Read the model definition and answer for the solid it produces. Units are mm, in the model's axes. A direction names the side the tool comes from. Coordinates: 2 decimals unless noted, no trailing zeros. Order: outer loops, then holes, each group sorted by start corner. A loop starts at its lowest first (then second) coordinate and runs counter-clockwise, first axis right, second up. Notation, with made-up numbers: (48, 87) - (83, 87) arc R28 cw to (83, 118) - close; hole circle Ø5 at (43.5, 50). An arc over 180 degrees is marked (long way). Write item = value, one per line.
from build123d import *

# Parameters (mm, degrees)
SKETCH1_W              = 140
SKETCH1_H              = 35
BOSS_EXTRUDE1_DEPTH    = 6
SKETCH2_R              = 4.5
SKETCH2_R_2            = 5.1
CUT_EXTRUDE1_DEPTH     = 7
CUT_EXTRUDE2_DEPTH     = 7
SKETCH234_W            = 10
SKETCH234_H            = 6
BOSS_EXTRUDE234_DEPTH  = 6
FILLET134_R            = 1
SKETCH2341_W           = 10
SKETCH2341_H           = 6
BOSS_EXTRUDE2341_DEPTH = 6
FILLET1341_R           = 1
SKETCH2342_W           = 10
SKETCH2342_H           = 6
BOSS_EXTRUDE2342_DEPTH = 6
FILLET1342_R           = 1
SKETCH2343_W           = 10
SKETCH2343_H           = 6
BOSS_EXTRUDE2343_DEPTH = 6
FILLET1343_R           = 1
SKETCH2344_W           = 10
SKETCH2344_H           = 6
BOSS_EXTRUDE2344_DEPTH = 6
FILLET1344_R           = 1
SKETCH2345_W           = 10
SKETCH2345_H           = 6
BOSS_EXTRUDE2345_DEPTH = 6
FILLET1345_R           = 1
SKETCH2346_W           = 10
SKETCH2346_H           = 6
BOSS_EXTRUDE2346_DEPTH = 6
FILLET1346_R           = 1
SKETCH2347_W           = 10
SKETCH2347_H           = 6
BOSS_EXTRUDE2347_DEPTH = 6
FILLET1347_R           = 1
SKETCH6_W              = 10
SKETCH6_H              = 6
CUT_EXTRUDE11_DEPTH    = 4
SKETCH61_W             = 10
SKETCH61_H             = 6
CUT_EXTRUDE12_DEPTH    = 4
SKETCH62_W             = 10
SKETCH62_H             = 6
CUT_EXTRUDE13_DEPTH    = 4
FILLET1348_R           = 5


with BuildPart() as part:
    # Sketch1 → Boss-Extrude1 (new body)
    with BuildSketch(Plane(origin=(0, 0, 0), x_dir=(1, 0, 0), z_dir=(0, 1, 0))):
        with Locations((70, 17.5)):
            Rectangle(SKETCH1_W, SKETCH1_H)
    extrude(amount=BOSS_EXTRUDE1_DEPTH)

    # Sketch2 → Cut-Extrude1 (cut, through all)
    with BuildSketch(Plane(origin=(0, 6, 0), x_dir=(1, 0, 0), z_dir=(0, 1, 0))):
        with Locations((66.4, 19)):
            Circle(SKETCH2_R)
        with Locations((35.4, 19)):
            Circle(SKETCH2_R_2)
    extrude(amount=-CUT_EXTRUDE1_DEPTH, mode=Mode.SUBTRACT)

    # Sketch3 → Cut-Extrude2 (cut, through all)
    with BuildSketch(Plane(origin=(0, 6, 0), x_dir=(1, 0, 0), z_dir=(0, 1, 0))):
        Polygon((140, 8), (100, 35), (140, 35), align=None)
    extrude(amount=-CUT_EXTRUDE2_DEPTH, mode=Mode.SUBTRACT)

    # Sketch234 → Boss-Extrude234 (add)
    with BuildSketch(Plane(origin=(119.232221392, 0, 0), x_dir=(1, 0, 0), z_dir=(0, 0, 1))):
        with Locations((0.767778608, 3)):
            Rectangle(SKETCH234_W, SKETCH234_H)
    extrude(amount=BOSS_EXTRUDE234_DEPTH)

    # Fillet134
    fillet134_edges = [part.edges().sort_by_distance(p)[0] for p in [
        (115, 3, 6),
        (125, 3, 6),
    ]]
    fillet(fillet134_edges, radius=FILLET134_R)

    # Sketch2341 → Boss-Extrude2341 (add)
    with BuildSketch(Plane(origin=(85.898888059, 0, 0), x_dir=(1, 0, 0), z_dir=(0, 0, 1))):
        with Locations((0.767778608, 3)):
            Rectangle(SKETCH2341_W, SKETCH2341_H)
    extrude(amount=BOSS_EXTRUDE2341_DEPTH)

    # Fillet1341
    fillet1341_edges = [part.edges().sort_by_distance(p)[0] for p in [
        (91.666666667, 3, 6),
        (81.666666667, 3, 6),
    ]]
    fillet(fillet1341_edges, radius=FILLET1341_R)

    # Sketch2342 → Boss-Extrude2342 (add)
    with BuildSketch(Plane(origin=(52.565554726, 0, 0), x_dir=(1, 0, 0), z_dir=(0, 0, 1))):
        with Locations((0.767778608, 3)):
            Rectangle(SKETCH2342_W, SKETCH2342_H)
    extrude(amount=BOSS_EXTRUDE2342_DEPTH)

    # Fillet1342
    fillet1342_edges = [part.edges().sort_by_distance(p)[0] for p in [
        (58.333333333, 3, 6),
        (48.333333333, 3, 6),
    ]]
    fillet(fillet1342_edges, radius=FILLET1342_R)

    # Sketch2343 → Boss-Extrude2343 (add)
    with BuildSketch(Plane(origin=(19.232221392, 0, 0), x_dir=(1, 0, 0), z_dir=(0, 0, 1))):
        with Locations((0.767778608, 3)):
            Rectangle(SKETCH2343_W, SKETCH2343_H)
    extrude(amount=BOSS_EXTRUDE2343_DEPTH)

    # Fillet1343
    fillet1343_edges = [part.edges().sort_by_distance(p)[0] for p in [
        (25, 3, 6),
        (15, 3, 6),
    ]]
    fillet(fillet1343_edges, radius=FILLET1343_R)

    # Sketch2344 → Boss-Extrude2344 (add)
    with BuildSketch(Plane(origin=(84.232221392, 6, -35), x_dir=(1, 0, 0), z_dir=(0, 0, -1))):
        with Locations((0.767778608, 3)):
            Rectangle(SKETCH2344_W, SKETCH2344_H)
    extrude(amount=BOSS_EXTRUDE2344_DEPTH)

    # Fillet1344
    fillet1344_edges = [part.edges().sort_by_distance(p)[0] for p in [
        (80, 3, -41),
        (90, 3, -41),
    ]]
    fillet(fillet1344_edges, radius=FILLET1344_R)

    # Sketch2345 → Boss-Extrude2345 (add)
    with BuildSketch(Plane(origin=(60.898888059, 6, -35), x_dir=(1, 0, 0), z_dir=(0, 0, -1))):
        with Locations((0.767778608, 3)):
            Rectangle(SKETCH2345_W, SKETCH2345_H)
    extrude(amount=BOSS_EXTRUDE2345_DEPTH)

    # Fillet1345
    fillet1345_edges = [part.edges().sort_by_distance(p)[0] for p in [
        (66.666666667, 3, -41),
        (56.666666667, 3, -41),
    ]]
    fillet(fillet1345_edges, radius=FILLET1345_R)

    # Sketch2346 → Boss-Extrude2346 (add)
    with BuildSketch(Plane(origin=(37.565554726, 6, -35), x_dir=(1, 0, 0), z_dir=(0, 0, -1))):
        with Locations((0.767778608, 3)):
            Rectangle(SKETCH2346_W, SKETCH2346_H)
    extrude(amount=BOSS_EXTRUDE2346_DEPTH)

    # Fillet1346
    fillet1346_edges = [part.edges().sort_by_distance(p)[0] for p in [
        (43.333333333, 3, -41),
        (33.333333333, 3, -41),
    ]]
    fillet(fillet1346_edges, radius=FILLET1346_R)

    # Sketch2347 → Boss-Extrude2347 (add)
    with BuildSketch(Plane(origin=(14.232221392, 6, -35), x_dir=(1, 0, 0), z_dir=(0, 0, -1))):
        with Locations((0.767778608, 3)):
            Rectangle(SKETCH2347_W, SKETCH2347_H)
    extrude(amount=BOSS_EXTRUDE2347_DEPTH)

    # Fillet1347
    fillet1347_edges = [part.edges().sort_by_distance(p)[0] for p in [
        (20, 3, -41),
        (10, 3, -41),
    ]]
    fillet(fillet1347_edges, radius=FILLET1347_R)

    # Sketch6 → Cut-Extrude11 (cut, symmetric)
    with BuildSketch(Plane(origin=(84.932221392, 3, -55), x_dir=(1, 0, 0), z_dir=(0, 1, 0))):
        with Locations((0.767778608, -44)):
            Rectangle(SKETCH6_W, SKETCH6_H)
    cut_extrude11 = extrude(amount=CUT_EXTRUDE11_DEPTH, both=True, mode=Mode.SUBTRACT)

    # Sketch61 → Cut-Extrude12 (cut, symmetric)
    with BuildSketch(Plane(origin=(53.132221392, 3, -55), x_dir=(1, 0, 0), z_dir=(0, 1, 0))):
        with Locations((0.767778608, -44)):
            Rectangle(SKETCH61_W, SKETCH61_H)
    cut_extrude12 = extrude(amount=CUT_EXTRUDE12_DEPTH, both=True, mode=Mode.SUBTRACT)

    # Sketch62 → Cut-Extrude13 (cut, symmetric)
    with BuildSketch(Plane(origin=(11.432221392, 3, -55), x_dir=(1, 0, 0), z_dir=(0, 1, 0))):
        with Locations((0.767778608, -44)):
            Rectangle(SKETCH62_W, SKETCH62_H)
    cut_extrude13 = extrude(amount=CUT_EXTRUDE13_DEPTH, both=True, mode=Mode.SUBTRACT)

    # Mirror1: Cut-Extrude11, Cut-Extrude12, Cut-Extrude13 across plane
    add(cut_extrude11.mirror(Plane.XY.offset(-19)), mode=Mode.SUBTRACT)
    add(cut_extrude12.mirror(Plane.XY.offset(-19)), mode=Mode.SUBTRACT)
    add(cut_extrude13.mirror(Plane.XY.offset(-19)), mode=Mode.SUBTRACT)

    # Fillet1348
    fillet1348_edges = [part.edges().sort_by_distance(p)[0] for p in [
        (140, 3, -8),
    ]]
    fillet(fillet1348_edges, radius=FILLET1348_R)


solid = part.part
1) Flat-ended cylindrical pins translate along their axes: pin 1 Ø2 at (x, y) = (96.5, 4) entering from -Z; pin 2 Ø3 at (y, z) = (2, -10.5) entering from +X; pin 3 Ø1.5 at (y, z) = (3.5, 1.5) entering from -X. Find the tip coordinate at first contact, or state that the pin passes through.
Returned:
pin_1 = -35
pin_2 = 138.41
pin_3 = 15
2) Determine the mould class of faces 1 (the face through (53, 3, 6)), 2 (the face through (12, 3, -24)), 3 (the face through (15, 3, 2)) for opening direction X: pulls with the +X half, pulls with the -X half, needs draft (parallel to the pull), parting line crosses it, or undercut.
Returned:
face_1 = needs draft
face_2 = undercut
face_3 = pulls with the -X half
3) For faces 4 (the face through (5, 3, -35)), 5 (the face through (66.667, 3, -37)), 6 (the face through (48.9, 3, -27)), 7 (the face through (7, 3, 0)), determine the directions among +Z, -Z, +X, -X, +Y, -Y from which every point of the face is accessible in a straight line to the end or side of a thin tool.
Returned:
face_4 = -Z, -X, +Y, -Y
face_5 = -Z, +Y, -Y
face_6 = +Y, -Y
face_7 = +Z, -X, +Y, -Y
4) The part is cut by section A-A (x = 51). Determine the outline of the cut face in (y, z), and give its area (3 significant figures).
Returned:
outline = (0, -35) - (6, -35) - (6, -30) - (0, -30) - close; (0, -24) - (6, -24) - (6, -14) - (0, -14) - close; (0, -8) - (6, -8) - (6, 6) - (0, 6) - close
area = 174 mm^2
5) The part is cut by section D-D (y = 1.75). Count the separate pieces of the cut face and the enclosed holes in it, and give its area (3 significant figures).
Returned:
separate_pieces = 1
enclosed_holes = 8
area = 4,330 mm^2
6) The part is cut by section C-C (z = -19). Determine the outline of the cut face in (x, y), and give its area (3 significant figures).
Returned:
outline = (0, 0) - (30.3, 0) - (30.3, 6) - (0, 6) - close; (40.5, 0) - (61.9, 0) - (61.9, 6) - (40.5, 6) - close; (70.9, 0) - (123.7, 0) - (123.7, 6) - (70.9, 6) - close
area = 627 mm^2
7) Straight lines are drawn through the part: line 1 along Z through (x, y) = (85.5, 3.75); line 2 along X through (y, z) = (1.25, 4.5); line 3 along Z through (x, y) = (35.4, 3.5). For each, find the intervals that lie inside material, in ascending order. Write a range as from..to.
Returned:
line_1 = -41..-30, -24..-14, -8..6
line_2 = 15..25, 48.33..58.33, 81.67..91.67, 115..125
line_3 = -41..-24.1, -13.9..0
8) The part is cut by section B-B (z = 1.5). Determine the outline of the cut face in (x, y).
Returned:
outline = (15, 0) - (25, 0) - (25, 6) - (15, 6) - close; (48.33, 0) - (58.33, 0) - (58.33, 6) - (48.33, 6) - close; (81.67, 0) - (91.67, 0) - (91.67, 6) - (81.67, 6) - close; (115, 0) - (125, 0) - (125, 6) - (115, 6) - close
